Geometry check sheet. Reference: the model listing, model coordinates, mm. Face numbers are marked on the shaded views. Round coordinates to 2 decimals unless told otherwise and drop trailing zeros. Order: outer loops, then holes, each group sorted by start corner. A loop starts at its lowest first (then second) coordinate and runs counter-clockwise, first axis right, second up. Notation, with made-up numbers: (-5, 71) - (14, 71) arc R12 cw to (14, 90) - close; hole circle Ø9 at (-18, 23.25). An arc over 180 degrees is marked (long way). Use a Markdown table: item, result. Add a question column.
(1) Gauge pin test, flat end, axial feed: P1, Ø2, axis at x = 0, y = 0, coming from the -Z side. Record the tip position at first contact, or that the pin passes through.
(2) Section check A-A on z = 0.95. Record the boundary of the cut face in (x, y), then the cut area to 3 significant figures.
(3) Thickness scan on line 1 along Y through (x, z) = (-0.65, 1.95); line 2 along X through (y, z) = (-0.5, 0.9); line 3 along Y through (x, z) = (0.9, 0.4). Record the ranges inside material, lowest first. Write a range as [from, to].
(4) Mould release check, pull along X, two halves, no side actions. Record for the marked faces 1, 2 and 3: released by +X, released by -X, zero draft, split by the parting line, or undercut.
```python
from build123d import *

# Parameters (mm, degrees)
F0_R     = 1.23
F1_DEPTH = 2.4
F4_SIZE  = 0.3


with BuildPart() as f1:
    # F0 (on Top) → F1 (new body)
    with BuildSketch(Plane.XY):
        Polygon((2.75, -1.587713), (2.75, 1.587713), (0, 3.175426), (-2.75, 1.587713), (-2.75, -1.587713), (0, -3.175426), align=None)
        Circle(F0_R, mode=Mode.SUBTRACT)
    extrude(amount=F1_DEPTH)

    # F2 (on Front) → F3 (revolve, cut)
    with BuildSketch(Plane.XZ):
        Polygon((4.828461, 0), (4.828461, 1.2), (2.75, 0), align=None)
        Polygon((4.828461, 2.4), (2.75, 2.4), (4.828461, 1.2), align=None)
    revolve(axis=Axis((0, 0, 1.176549), (0, 0, 1)), mode=Mode.SUBTRACT)

    # F4
    f4_edges = [f1.edges().sort_by_distance(p)[0] for p in [
        (1.23, 0, 1.2),
        (-1.23, 0, 0),
        (-1.23, 0, 2.4),
    ]]
    chamfer(f4_edges, length=F4_SIZE)


solid = f1.part
```
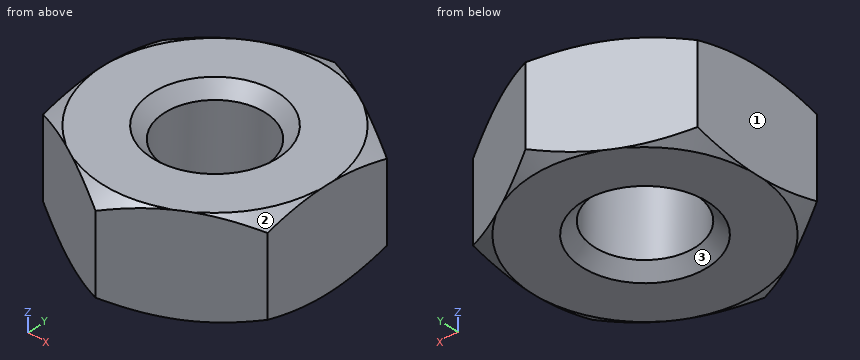
Check sheet entries:
| question | item | result |
|---|---|---|
| 1 | P1 | passes through |
| 2 | outline | (-2.75, -1.59) - (0, -3.18) - (2.75, -1.59) - (2.75, 1.59) - (0, 3.18) - (-2.75, 1.59) - close; hole circle Ø2.46 at (0, 0) |
| 2 | area | 21.4 mm2 |
| 3 | line 1 | y = [-2.8, -1.04], [1.04, 2.8] |
| 3 | line 2 | x = [-2.75, -1.12], [1.12, 2.75] |
| 3 | line 3 | y = [-2.66, -0.84], [0.84, 2.66] |
| 4 | face 1 | released by -X |
| 4 | face 2 | released by +X |
| 4 | face 3 | undercut |
